Could you check a few things on this drawing? It's one solid part, dimensions in mm from its lowest x, y, z. Round coordinates to 2 decimals unless told otherwise and drop trailing zeros. Order: outer loops, then holes, each group sorted by start corner. A loop starts at its lowest first (then second) coordinate and runs counter-clockwise, first axis right, second up. Notation, with made-up numbers: (80.5, -30) -> (135.5, -30) arc R28 cw to (135.5, -4) -> close; hole circle Ø11 at (-35.75, 89.5). An arc over 180 degrees is marked (long way). Use a Markdown table: item, result. Add a question column.
(1) If I drill on probe 1 along X at (y, z) = (17, 5.5); probe 2 along X at (y, z) = (18.5, 13.75); probe 3 along Y at (x, z) = (7.5, 13.5), over which ranges is the centre line in solid material (lowest first)?
(2) I want a section at A-A, the plane z = 12.25. Please give me the cut outline in (x, y).
(3) I'm going to push flat-ended pins straight in: P1, Ø8, axis at x = 10, z = 8.5, coming from the +Y side; P2, Ø8, axis at y = 16.5, z = 4, coming from the +X side; P3, Ø1.5, axis at x = 6.5, z = 5, coming from the -Y side; P4, Ø2, axis at y = 30.5, z = 8.5, coming from the -X side. Where does each tip first touch, or does it pass through?
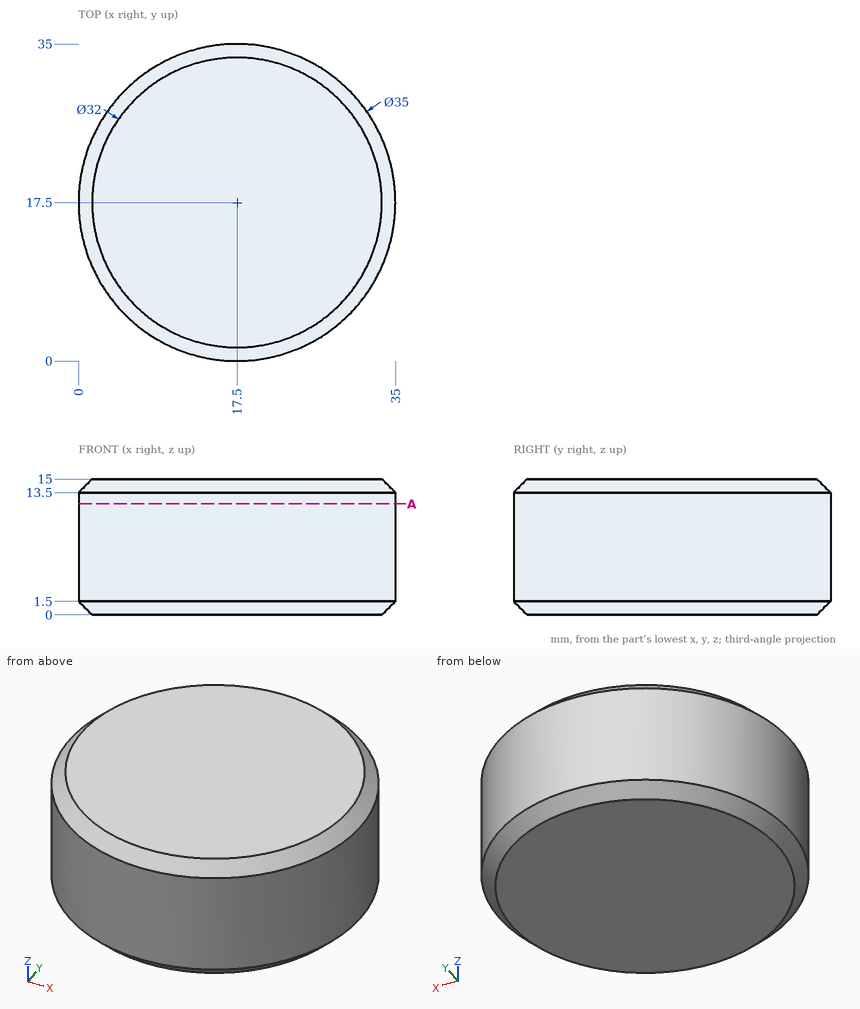
Taken from the geometry:
| question | item | result |
|---|---|---|
| 1 | probe 1 | x = 0.01 to 34.99 |
| 1 | probe 2 | x = 0.28 to 34.72 |
| 1 | probe 3 | y = 3.14 to 31.86 |
| 2 | outline | circle Ø35 at (17.5, 17.5) |
| 3 | P1 | stops at y = 34.65 |
| 3 | P2 | stops at x = 35 |
| 3 | P3 | stops at y = 3.32 |
| 3 | P4 | stops at x = 4.76 |
